```python
from build123d import *

# Parameters (mm, degrees)
SKETCH010_AS_DRAWN_R                      = 3
EXTRUDE009_DEPTH                          = 40
EXTRUDE009_ONTO_SKETCH010_PLACEMENT_ANGLE = 9
EXTRUDE001_DEPTH                          = 5
EXTRUDE001_PLACEMENT_ANGLE                = 45


with BuildPart() as extrude009:
    # Sketch010 as drawn → Extrude009 (new)
    with BuildSketch(Plane.XY):
        Circle(SKETCH010_AS_DRAWN_R)
    extrude(amount=-EXTRUDE009_DEPTH)


with BuildPart() as extrude009_1:
    # Extrude009 onto Sketch010 placement: moved
    add(extrude009.part.moved(Location((-32, -32, 30))).rotate(Axis((-32, -32, 30), (0, 0, -1)), EXTRUDE009_ONTO_SKETCH010_PLACEMENT_ANGLE))


with BuildPart() as cut003:
    # Sketch001 (on Face7 of Extrude) → Extrude001 (new body)
    with BuildSketch(Plane(origin=(0, 0, 0), x_dir=(1, 0, 0), z_dir=(0, 0, -1))):
        with BuildLine():
            Line((20, 0), (20, 110))
            Line((20, 110), (-20, 110))
            Line((-20, 110), (-20, 0))
            ThreePointArc((20, 0), (0, 20), (-20, 0))
        make_face()
    extrude(amount=-EXTRUDE001_DEPTH)


with BuildPart() as cut003_1:
    # Extrude001 placement: moved
    add(cut003.part.rotate(Axis((0, 0, 0), (0, 0, -1)), EXTRUDE001_PLACEMENT_ANGLE))

    # Cut003: cut Extrude009
    add(extrude009_1.part, mode=Mode.SUBTRACT)


solid = cut003_1.part
```
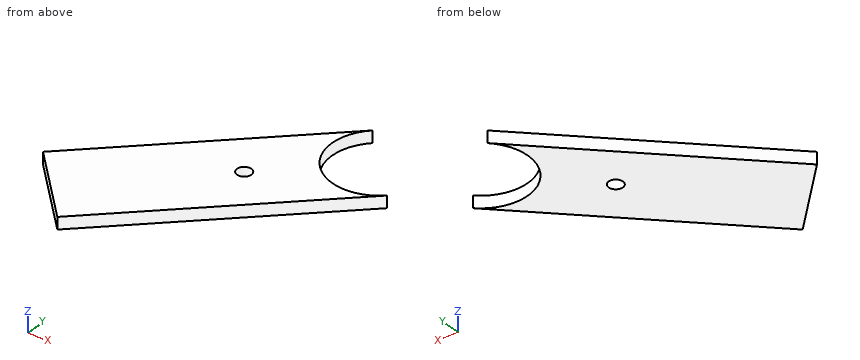
Design review of the part built by this model. Coordinates are the model's own, in mm. Coordinates: 2 decimals unless noted, no trailing zeros. Loops run counter-clockwise (first coordinate to the right, second up) from the corner with the lowest first, then second, coordinate; pieces in that order, holes last. Notation, with made-up numbers: (30.25, 27) - (82.25, 27) arc R22 cw to (82.25, 42) - close; hole circle Ø11 at (88.25, 25.25). An arc over 180 degrees is marked (long way). Use CSV: the item, a comma, the result in double quotes. Start each with the question number.
1) Consider section A-A on x = -32. Write out the cut boundary in (y, z).
2) Wall thickness on L1, parallel to Y at x = -32, z = 1.6; L2, parallel to X at y = -67, z = 0.7: over which ranges is each line inside the solid? List them lowest first. Write a range as from..to.
3) For pin 1 Ø3 at (y, z) = (-2.5, 2.5) entering from -X; pin 2 Ø1 at (y, z) = (-19.5, 1.5) entering from +X, all flat-tipped, find the tip position at first contact; note any pin that passes through.
4) Consider section B-B on z = 1.25. Write out the cut boundary in (x, y), then the cut area to 3 significant figures.
5) Consider section D-D on x = -76.5. Write out the cut boundary in (y, z).
6) Consider section C-C on y = -3. Write out the cut boundary in (x, z).
Geometry says:
1,outline,"(-60.28, 0) - (-35, 0) - (-35, 5) - (-60.28, 5) - close; (-29, 0) - (-3.72, 0) - (-3.72, 5) - (-29, 5) - close"
2,L1,"-60.28..-35, -29..-3.72"
2,L2,"-88.56..-38.72"
3,pin 1,"x = -32.28"
3,pin 2,"x = 9.28"
4,outline,"(-91.92, -63.64) - (-63.64, -91.92) - (14.14, -14.14) arc R20 cw to (-14.14, 14.14) - close; hole circle Ø6 at (-32, -32)"
4,area,"3,740 mm^2"
5,outline,"(-79.06, 0) - (-48.22, 0) - (-48.22, 5) - (-79.06, 5) - close"
6,outline,"(-31.28, 0) - (-19.77, 0) - (-19.77, 5) - (-31.28, 5) - close"
